The model under review builds one solid part; all positions refer to its coordinate system, in mm. Coordinates: 2 decimals unless noted, no trailing zeros. Order: outer loops, then holes, each group sorted by start corner. A loop starts at its lowest first (then second) coordinate and runs counter-clockwise, first axis right, second up. Notation, with made-up numbers: (63.5, 82) -> (71.5, 82) arc R15 ccw to (71.5, 90) -> close; hole circle Ø8 at (65.5, 19). An arc over 180 degrees is marked (long way). Use one line per item in the form item = value. Start each with the question number.
(1) Take a section at D-D (y = -11). State the section outline as (x, z) points, then the cut area to 3 significant figures.
(2) Take a section at B-B (x = 0). State the section outline as (y, z) points.
(3) Wall thickness on line 1 along X through (y, z) = (-31, 0.85); line 2 along Y through (x, z) = (-13, 1.3); line 3 along Y through (x, z) = (-63.5, 1.5): over which ranges is each line inside the solid? List them lowest first.
(4) Insertion check: pin 1 Ø1.9 at (x, y) = (-63.5, 42.75) entering from +Z. The pin has a flat end and moves straight along its axis. Give the tip position at first contact, or say it passes through.
(5) Take a section at C-C (z = 0.6). State how many separate pieces and enclosed holes the cut face has, then the cut area to 3 significant figures.
(6) Take a section at A-A (y = -29.5). State the section outline as (x, z) points, then the cut area to 3 significant figures.
```python
from build123d import *

# Parameters (mm, degrees)
SKETCH_W        = 133
SKETCH_H        = 91.5
SKETCH_R        = 1.6
PAD_DEPTH       = 2
SKETCH001_R     = 1.7
POCKET_DEPTH    = 2.001
POCKET001_DEPTH = 2.001
FILLET_R        = 2.5


with BuildPart() as part:
    # Sketch → Pad (new body)
    with BuildSketch(Plane.XY):
        Rectangle(SKETCH_W, SKETCH_H)
        with Locations((-63.5, 42.75)):
            Circle(SKETCH_R, mode=Mode.SUBTRACT)
        with Locations((0, 42.75)):
            Circle(SKETCH_R, mode=Mode.SUBTRACT)
        with Locations((63.5, 42.75)):
            Circle(SKETCH_R, mode=Mode.SUBTRACT)
        with Locations((0, -42.75)):
            Circle(SKETCH_R, mode=Mode.SUBTRACT)
        with Locations((63.5, -42.75)):
            Circle(SKETCH_R, mode=Mode.SUBTRACT)
        with Locations((-63.5, -42.75)):
            Circle(SKETCH_R, mode=Mode.SUBTRACT)
    extrude(amount=PAD_DEPTH)

    # Sketch001 (on Face12 of Pad) → Pocket (cut, through all)
    with BuildSketch(Plane.XY.offset(2)):
        with Locations((13, 0)):
            Circle(SKETCH001_R)
        with Locations((53.5, 0)):
            Circle(SKETCH001_R)
        with Locations((-13, 0)):
            Circle(SKETCH001_R)
        with Locations((-53.5, 0)):
            Circle(SKETCH001_R)
    extrude(amount=-POCKET_DEPTH, mode=Mode.SUBTRACT)

    # Sketch002 (on Face5 of Pocket) → Pocket001 (cut, through all)
    with BuildSketch(Plane.XY.offset(2)):
        with BuildLine():
            Line((-59, 38.25), (-59, 8.25))
            ThreePointArc((-59, 8.25), (-58.267767, 6.482233), (-56.5, 5.75))
            Line((-56.5, 5.75), (-44, 5.75))
            ThreePointArc((-44, 5.75), (-42.700268, 6.114421), (-41.779456, 7.101443))
            Line((-41.779456, 7.101443), (-34.279456, 21.601443))
            ThreePointArc((-34.279456, 21.601443), (-34.070868, 22.158967), (-34, 22.75))
            Line((-34, 22.75), (-34, 38.25))
            ThreePointArc((-34, 38.25), (-34.732233, 40.017767), (-36.5, 40.75))
            Line((-36.5, 40.75), (-56.5, 40.75))
            ThreePointArc((-56.5, 40.75), (-58.267767, 40.017767), (-59, 38.25))
        make_face()
        with BuildLine():
            Line((-28.5, 38.25), (-28.5, 22.75))
            ThreePointArc((-28.5, 22.75), (-28.429132, 22.158967), (-28.220544, 21.601443))
            Line((-28.220544, 21.601443), (-20.720544, 7.101443))
            ThreePointArc((-20.720544, 7.101443), (-19.799732, 6.114421), (-18.5, 5.75))
            Line((-18.5, 5.75), (-6, 5.75))
            ThreePointArc((-6, 5.75), (-4.232233, 6.482233), (-3.5, 8.25))
            Line((-3.5, 8.25), (-3.5, 38.25))
            ThreePointArc((-3.5, 38.25), (-4.232233, 40.017767), (-6, 40.75))
            Line((-6, 40.75), (-26, 40.75))
            ThreePointArc((-26, 40.75), (-27.767767, 40.017767), (-28.5, 38.25))
        make_face()
        with BuildLine():
            Line((59, -38.25), (59, -8.25))
            ThreePointArc((59, -8.25), (58.267767, -6.482233), (56.5, -5.75))
            Line((56.5, -5.75), (44, -5.75))
            ThreePointArc((44, -5.75), (42.700268, -6.114421), (41.779456, -7.101443))
            Line((41.779456, -7.101443), (34.279456, -21.601443))
            ThreePointArc((34.279456, -21.601443), (34.070868, -22.158967), (34, -22.75))
            Line((34, -22.75), (34, -38.25))
            ThreePointArc((34, -38.25), (34.732233, -40.017767), (36.5, -40.75))
            Line((36.5, -40.75), (56.5, -40.75))
            ThreePointArc((56.5, -40.75), (58.267767, -40.017767), (59, -38.25))
        make_face()
        with BuildLine():
            Line((28.5, -38.25), (28.5, -22.75))
            ThreePointArc((28.5, -22.75), (28.429132, -22.158967), (28.220544, -21.601443))
            Line((28.220544, -21.601443), (20.720544, -7.101443))
            ThreePointArc((20.720544, -7.101443), (19.799732, -6.114421), (18.5, -5.75))
            Line((18.5, -5.75), (6, -5.75))
            ThreePointArc((6, -5.75), (4.232233, -6.482233), (3.5, -8.25))
            Line((3.5, -8.25), (3.5, -38.25))
            ThreePointArc((3.5, -38.25), (4.232233, -40.017767), (6, -40.75))
            Line((6, -40.75), (26, -40.75))
            ThreePointArc((26, -40.75), (27.767767, -40.017767), (28.5, -38.25))
        make_face()
        with BuildLine():
            Line((59, 38.25), (59, 8.25))
            ThreePointArc((56.5, 5.75), (58.267767, 6.482233), (59, 8.25))
            Line((56.5, 5.75), (44, 5.75))
            ThreePointArc((41.779456, 7.101443), (42.700268, 6.114421), (44, 5.75))
            Line((41.779456, 7.101443), (34.279456, 21.601443))
            ThreePointArc((34, 22.75), (34.070868, 22.158967), (34.279456, 21.601443))
            Line((34, 22.75), (34, 38.25))
            ThreePointArc((36.5, 40.75), (34.732233, 40.017767), (34, 38.25))
            Line((36.5, 40.75), (56.5, 40.75))
            ThreePointArc((59, 38.25), (58.267767, 40.017767), (56.5, 40.75))
        make_face()
        with BuildLine():
            Line((28.5, 38.25), (28.5, 22.75))
            ThreePointArc((28.220544, 21.601443), (28.429132, 22.158967), (28.5, 22.75))
            Line((28.220544, 21.601443), (20.720544, 7.101443))
            ThreePointArc((18.5, 5.75), (19.799732, 6.114421), (20.720544, 7.101443))
            Line((18.5, 5.75), (6, 5.75))
            ThreePointArc((3.5, 8.25), (4.232233, 6.482233), (6, 5.75))
            Line((3.5, 8.25), (3.5, 38.25))
            ThreePointArc((6, 40.75), (4.232233, 40.017767), (3.5, 38.25))
            Line((6, 40.75), (26, 40.75))
            ThreePointArc((28.5, 38.25), (27.767767, 40.017767), (26, 40.75))
        make_face()
        with BuildLine():
            Line((-59, -38.25), (-59, -8.25))
            ThreePointArc((-56.5, -5.75), (-58.267767, -6.482233), (-59, -8.25))
            Line((-56.5, -5.75), (-44, -5.75))
            ThreePointArc((-41.779456, -7.101443), (-42.700268, -6.114421), (-44, -5.75))
            Line((-41.779456, -7.101443), (-34.279456, -21.601443))
            ThreePointArc((-34, -22.75), (-34.070868, -22.158967), (-34.279456, -21.601443))
            Line((-34, -22.75), (-34, -38.25))
            ThreePointArc((-36.5, -40.75), (-34.732233, -40.017767), (-34, -38.25))
            Line((-36.5, -40.75), (-56.5, -40.75))
            ThreePointArc((-59, -38.25), (-58.267767, -40.017767), (-56.5, -40.75))
        make_face()
        with BuildLine():
            Line((-28.5, -38.25), (-28.5, -22.75))
            ThreePointArc((-28.220544, -21.601443), (-28.429132, -22.158967), (-28.5, -22.75))
            Line((-28.220544, -21.601443), (-20.720544, -7.101443))
            ThreePointArc((-18.5, -5.75), (-19.799732, -6.114421), (-20.720544, -7.101443))
            Line((-18.5, -5.75), (-6, -5.75))
            ThreePointArc((-3.5, -8.25), (-4.232233, -6.482233), (-6, -5.75))
            Line((-3.5, -8.25), (-3.5, -38.25))
            ThreePointArc((-6, -40.75), (-4.232233, -40.017767), (-3.5, -38.25))
            Line((-6, -40.75), (-26, -40.75))
            ThreePointArc((-28.5, -38.25), (-27.767767, -40.017767), (-26, -40.75))
        make_face()
    extrude(amount=-POCKET001_DEPTH, mode=Mode.SUBTRACT)

    # Fillet
    fillet_edges = [part.edges().sort_by_distance(p)[0] for p in [
        (-66.5, -45.75, 1),
        (66.5, -45.75, 1),
        (66.5, 45.75, 1),
        (-66.5, 45.75, 1),
    ]]
    fillet(fillet_edges, radius=FILLET_R)


solid = part.part
```
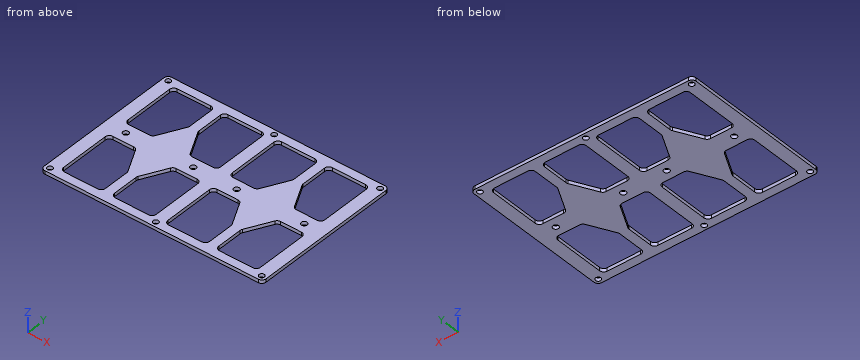
Findings:
q1.outline = (-66.5, 0) -> (-59, 0) -> (-59, 2) -> (-66.5, 2) -> close; (-39.76, 0) -> (-22.74, 0) -> (-22.74, 2) -> (-39.76, 2) -> close; (-3.5, 0) -> (3.5, 0) -> (3.5, 2) -> (-3.5, 2) -> close; (22.74, 0) -> (39.76, 0) -> (39.76, 2) -> (22.74, 2) -> close; (59, 0) -> (66.5, 0) -> (66.5, 2) -> (59, 2) -> close
q1.area = 112 mm²
q2.outline = (-45.75, 0) -> (-44.35, 0) -> (-44.35, 2) -> (-45.75, 2) -> close; (-41.15, 0) -> (41.15, 0) -> (41.15, 2) -> (-41.15, 2) -> close; (44.35, 0) -> (45.75, 0) -> (45.75, 2) -> (44.35, 2) -> close
q3.line_1 = -66.5 to -59, -34 to -28.5, -3.5 to 3.5, 28.5 to 34, 59 to 66.5
q3.line_2 = -45.75 to -40.75, -5.75 to -1.7, 1.7 to 5.75, 40.75 to 45.75
q3.line_3 = -45.75 to -44.35, -41.15 to 41.15, 44.35 to 45.75
q4.pin_1 = through
q5.separate_pieces = 1
q5.enclosed_holes = 18
q5.area = 5,670 mm²
q6.outline = (-66.5, 0) -> (-59, 0) -> (-59, 2) -> (-66.5, 2) -> close; (-34, 0) -> (-28.5, 0) -> (-28.5, 2) -> (-34, 2) -> close; (-3.5, 0) -> (3.5, 0) -> (3.5, 2) -> (-3.5, 2) -> close; (28.5, 0) -> (34, 0) -> (34, 2) -> (28.5, 2) -> close; (59, 0) -> (66.5, 0) -> (66.5, 2) -> (59, 2) -> close
q6.area = 66.0 mm²
